Verification items for this drawing (mm, ordinates from the low corner). Round coordinates to 2 decimals unless told otherwise and drop trailing zeros. Loops run counter-clockwise (first coordinate to the right, second up) from the corner with the lowest first, then second, coordinate; pieces in that order, holes last. Notation, with made-up numbers: (67, 69) -> (126, 69) arc R34 cw to (126, 100) -> close; hole circle Ø6 at (-36, -26.5). An arc over 180 degrees is marked (long way). Use a Markdown table: item, result. Add a question column.
Q1. Sectioned sample at C-C, the plane z = 27. Enter the section's corners in (x, y), then the cut area to 3 significant figures.
Q2. Sectioned sample at A-A, the plane x = 3. Enter the section's corners in (y, z), then the cut area to 3 significant figures.
Q3. Sectioned sample at D-D, the plane x = 0.8. Enter the section's corners in (y, z), then the cut area to 3 significant figures.
Q4. Release check for a two-part mould opening along Y. For the marked faces 1 and 2 record: released by +Y, released by -Y, zero draft, split by the parting line, or undercut.
Q5. Material ranges on L1, parallel to Y at x = 3, z = 28.5; L2, parallel to Z at x = 2.85, y = 2.1; L3, parallel to X at y = 2.75, z = 6.5, recorded low to high.
Q6. Gauge pin test, flat ends, axial feed: P1, Ø1.5, axis at x = 5, y = 4, coming from the -Z side; P2, Ø3, axis at x = 3, y = 3, coming from the -Z side; P3, Ø1.5, axis at x = 5, z = 9, coming from the -Y side; P4, Ø1.6, axis at x = 3, y = 2.5, coming from the +Z side. Record the tip position at first contact, or that the pin passes through.
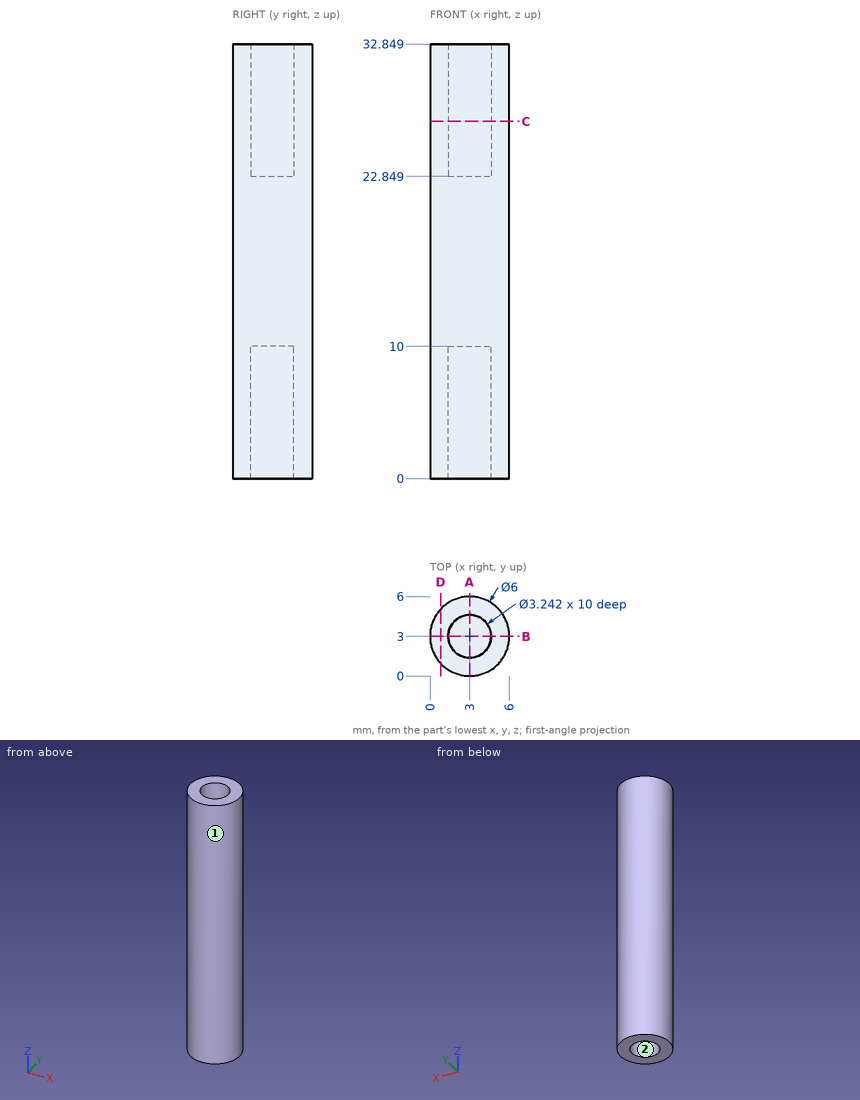
Values:
| question | item | result |
|---|---|---|
| 1 | outline | circle Ø6 at (3, 3); hole circle Ø3.24 at (3, 3) |
| 1 | area | 20.0 mm^2 |
| 2 | outline | (0, 0) -> (1.38, 0) -> (1.38, 10) -> (4.62, 10) -> (4.62, 0) -> (6, 0) -> (6, 32.85) -> (4.62, 32.85) -> (4.62, 22.85) -> (1.38, 22.85) -> (1.38, 32.85) -> (0, 32.85) -> close |
| 2 | area | 132 mm^2 |
| 3 | outline | (0.96, 0) -> (5.04, 0) -> (5.04, 32.85) -> (0.96, 32.85) -> close |
| 3 | area | 134 mm^2 |
| 4 | face 1 | split by the parting line |
| 4 | face 2 | undercut |
| 5 | L1 | 0 to 1.38, 4.62 to 6 |
| 5 | L2 | 10 to 22.85 |
| 5 | L3 | 0.01 to 1.4, 4.6 to 5.99 |
| 6 | P1 | z = 0 |
| 6 | P2 | z = 10 |
| 6 | P3 | y = 0.27 |
| 6 | P4 | z = 22.85 |
